Source: three-view drawing plus pictorial views. Frame: mm from the lowest corner of the part. A direction names the side the tool comes from. Coordinates: 2 decimals unless noted, no trailing zeros. Order: outer loops, then holes, each group sorted by start corner. A loop starts at its lowest first (then second) coordinate and runs counter-clockwise, first axis right, second up. Notation, with made-up numbers: (17.5, 59.5) - (25.5, 59.5) arc R15 ccw to (25.5, 63.5) - close; hole circle Ø2 at (-29, -4). An arc over 180 degrees is marked (long way). One line per question, with ' | ' between items.
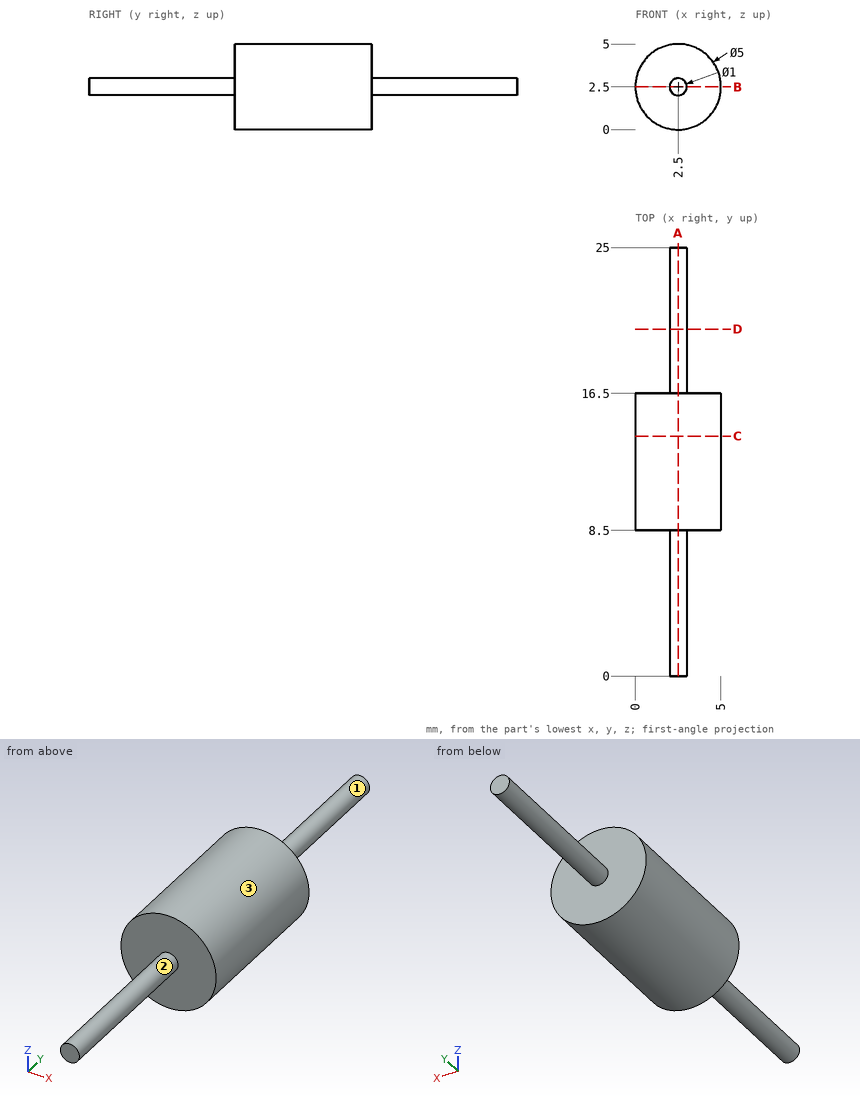
Item 1: Section B-B on z = 2.5. Return the cut outline in (x, y).
Data:
outline: (0, 8.5) - (2, 8.5) - (2, 0) - (3, 0) - (3, 8.5) - (5, 8.5) - (5, 16.5) - (3, 16.5) - (3, 25) - (2, 25) - (2, 16.5) - (0, 16.5) - close
Item 2: Section A-A on x = 2.5. Return the cut outline in (y, z).
Data:
outline: (0, 2) - (8.5, 2) - (8.5, 0) - (16.5, 0) - (16.5, 2) - (25, 2) - (25, 3) - (16.5, 3) - (16.5, 5) - (8.5, 5) - (8.5, 3) - (0, 3) - close
Item 3: Contact query for flat-ended pins moving along their axis: P1, Ø1.5, axis at y = 3.5, z = 1.5, coming from the +X side; P2, Ø1.5, axis at y = 20, z = 2, coming from the -X side; P3, Ø1.5, axis at x = 1.5, z = 1.5, coming from the +Y side. Output: stop coordinate, or through.
Data:
P1: x = 2.93 | P2: x = 2 | P3: y = 16.5
Item 4: Ray query, line 1 (Y direction, x = 2.35, z = 1.1); line 2 (Z direction, x = 2.5, y = 17.5); line 3 (X direction, y = 1.5, z = 2.3). Return the intervals inside material, ascending.
Data:
line 1: 8.5 to 16.5 | line 2: 2 to 3 | line 3: 2.04 to 2.96
Item 5: Section C-C on y = 14. Return the cut outline in (x, z).
Data:
outline: circle Ø5 at (2.5, 2.5)
Item 6: Access query for the marked faces 1, 2 and 3. Directions: +Z, -Z, +X, -X, +Y, -Y. A direction counts if a zero-diameter tool reaches every point of the face in a straight line with its end or side. Return the directions, or none.
Data:
face 1: +Y | face 2: -Y | face 3: +Y, -Y
Item 7: Section D-D on y = 20.25. Return the cut outline in (x, z).
Data:
outline: circle Ø1 at (2.5, 2.5)
